For this review, use the dimensioned drawing (mm, ordinates from the lowest corner) and the shaded views. A direction names the side the tool comes from. Give positions to 0.01 mm unless a question says otherwise; leave off trailing zeros. Write each loop counter-clockwise with the first axis right and the second up, starting at its lowest first coordinate (ties: lowest second). Pieces come first, ordered by that corner, then holes.
1) Draft analysis for pull direction Y (two halves, no side actions). For the marked faces 5, 6 and 7, state which applies: pulls with the +Y half, pulls with the -Y half, needs draft (parallel to the pull), parting line crosses it, or undercut.
2) Wall thickness on line 1 along Y through (x, z) = (22.5, 1.7); line 2 along X through (y, z) = (23, 1) (1 decimal); line 3 along Z through (x, y) = (42, 32): over which ranges is each line inside the solid? List them lowest first.
3) We need section B-B on x = 5.5. Give the boundary of the cut face in (y, z), and give its area (3 significant figures).
4) For P1, Ø6, axis at x = 38.5, z = 3, coming from the +Y side (1 decimal); P2, Ø3.5, axis at x = 19.5, z = 8.5, coming from the -Y side; P3, Ø2, axis at x = 15.5, z = 4.5, coming from the +Y side, all flat-tipped, find the tip position at first contact; note any pin that passes through.
5) Machinability: for the marked faces 1, 2, 3 and 4, which of the approach directions +Z, -Z, +X, -X, +Y, -Y give a long, thin tool a straight path to every point of the face, cutting with its end or side? Answer none if there is none.
6) We need section C-C on z = 2.25. Give the boundary of the cut face in (x, y) (1 decimal).
7) We need section D-D on x = 22. Give the boundary of the cut face in (y, z) (1 decimal).
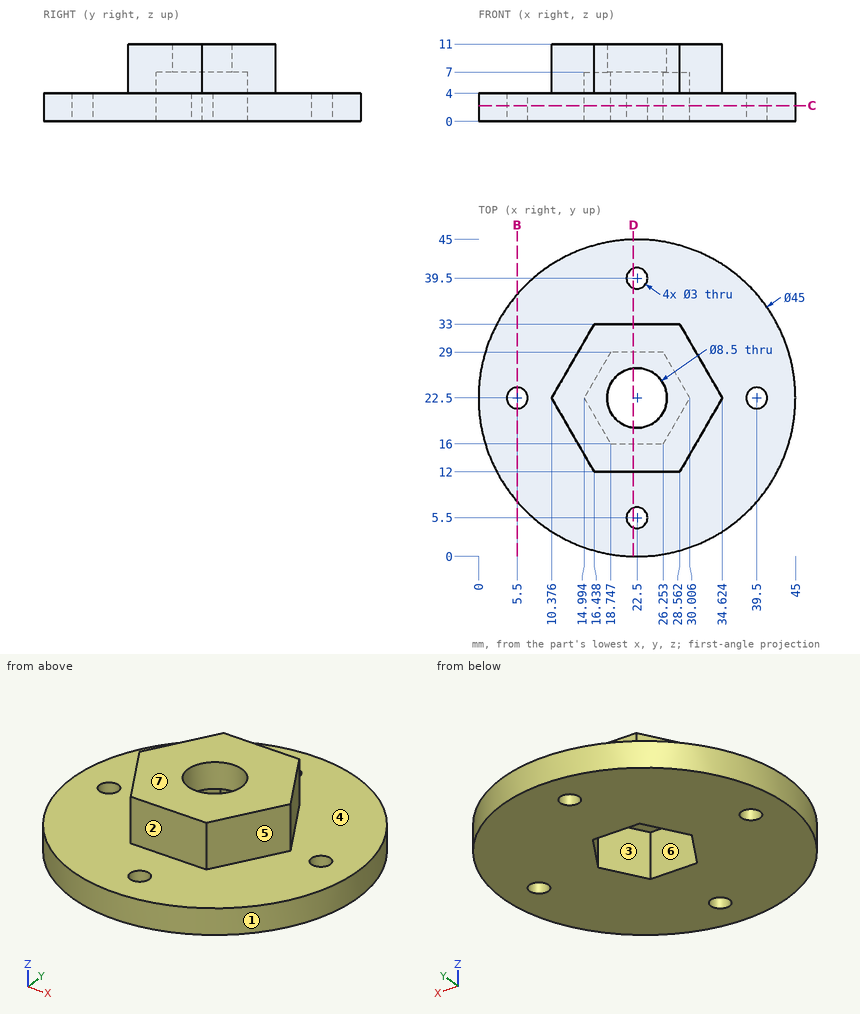
Results list:
1. face 5: pulls with the -Y half
1. face 6: undercut
1. face 7: needs draft
2. line 1: y = 0 to 4, 7 to 16, 29 to 38, 41 to 45
2. line 2: x = 0 to 4.1, 6.9 to 15.3, 29.7 to 38.1, 40.9 to 45
2. line 3: z = 0 to 4
3. outline: (7.76, 0) - (21, 0) - (21, 4) - (7.76, 4) - close; (24, 0) - (37.24, 0) - (37.24, 4) - (24, 4) - close
3. area: 106 mm2
4. P1: stops at y = 40.9
4. P2: stops at y = 12
4. P3: stops at y = 44.15
5. face 1: +Z, -Z
5. face 2: +Z, +X, -X, -Y
5. face 3: -Z
5. face 4: +Z
6. outline: circle Ø45 at (22.5, 22.5); hole circle Ø3 at (5.5, 22.5); hole (15, 22.5) - (18.7, 16) - (26.3, 16) - (30, 22.5) - (26.3, 29) - (18.7, 29) - close; hole circle Ø3 at (22.5, 5.5); hole circle Ø3 at (22.5, 39.5); hole circle Ø3 at (39.5, 22.5)
7. outline: (0, 0) - (4.1, 0) - (4.1, 4) - (0, 4) - close; (6.9, 0) - (16, 0) - (16, 7) - (18.3, 7) - (18.3, 11) - (12, 11) - (12, 4) - (6.9, 4) - close; (26.7, 7) - (29, 7) - (29, 0) - (38.1, 0) - (38.1, 4) - (33, 4) - (33, 11) - (26.7, 11) - close; (40.9, 0) - (45, 0) - (45, 4) - (40.9, 4) - close
